Read the model definition and answer for the solid it produces. Units are mm, in the model's axes. Face numbers are marked on the shaded views. A direction names the side the tool comes from. Give positions to 0.01 mm unless a question says otherwise; leave off trailing zeros. Order: outer loops, then holes, each group sorted by start corner. A loop starts at its lowest first (then second) coordinate and runs counter-clockwise, first axis right, second up. Notation, with made-up numbers: M 16.5,70 L 36.5,70 A12 cw 36.5,79 Z; hole C 74,37 d6. An arc over 180 degrees is marked long. One line per item, written item: value.
Autodesk Inventor part; units mm, degrees
ref_plane "YZ Plane" through (0, 0, 0) normal (1, 0, 0) x (0, 1, 0)
ref_plane "XZ Plane" through (0, 0, 0) normal (0, 1, 0) x (-1, 0, 0)
ref_plane "XY Plane" through (0, 0, 0) normal (0, 0, 1) x (1, 0, 0)
sketch "Boceto1" plane through (0, 0, 0) normal (0, 1, 0) x (-1, 0, 0)
  line L0 (0, 0) -> (640, 0)
  line L1 (640, 0) -> (640, 1009)
  line L2 (640, 1009) -> (0, 1009)
  line L3 (0, 1009) -> (0, 0)
  dimension "d0" = 640
  dimension "d1" = 1009
extrude "Extrusión1" add sketch "Boceto1" along normal blind 1147
sketch "Boceto2" plane through (0, 1147, 0) normal (0, 1, 0) x (1, 0, 0)
  line L0 (-640, 0) -> (-640, -1009) construction
  line L1 (-640, -1009) -> (0, -1009) construction
  line L2 (0, -1009) -> (0, 0) construction
  line L3 (0, 0) -> (-640, 0) construction
  line L4 (-640, 0) -> (-640, -1009) construction
  line L5 (-640, -1009) -> (-640, -504.5) construction
  line L6 (0, -1009) -> (0, 0) construction
  line L7 (-640, -504.5) -> (0, -504.5) construction
  line L8 (0, -504.5) -> (0, -434.5) construction
  line L9 (0, -434.5) -> (-640, -434.5) construction
  line L10 (-640, -434.5) -> (-640, -504.5) construction
  line L11 (0, -434.5) -> (-640, -434.5)
  line L12 (-640, -434.5) -> (-640, -504.5)
  line L13 (-640, -504.5) -> (0, -504.5)
  line L14 (0, -504.5) -> (0, -434.5)
  dimension "d4" = 504.5
  dimension "d5" = 70
  dimension "d6" = 70
extrude "Extrusión2" add sketch "Boceto2" along normal blind 633
sketch "Boceto3" plane through (0, 1147, 0) normal (0, 1, 0) x (1, 0, 0)
  line L0 (-640, -434.5) -> (0, -434.5) construction
  line L1 (0, -434.5) -> (0, 0) construction
  line L2 (0, 0) -> (-640, 0) construction
  line L3 (-640, 0) -> (-640, -434.5) construction
  line L4 (0, -434.5) -> (0, 0) construction
  line L5 (0, -434.5) -> (-160, -434.5) construction
  line L6 (0, -434.5) -> (-640, -434.5) construction
  line L7 (-640, -434.5) -> (-640, -504.5) construction
  line L8 (-640, -434.5) -> (-480, -434.5) construction
  line L9 (-480, -434.5) -> (-160, -434.5)
  line L10 (-160, -434.5) -> (-160, -134.5)
  line L11 (-160, -134.5) -> (-480, -134.5)
  line L12 (-480, -134.5) -> (-480, -434.5)
  dimension "d9" = 160
  dimension "d10" = 160
  dimension "d11" = 300
extrude "Extrusión3" add sketch "Boceto3" along normal blind 53
sketch "Boceto4" plane through (0, 1200, 0) normal (0, 1, 0) x (1, 0, 0)
  line L0 (-160, -434.5) -> (-480, -434.5) construction
  line L1 (-160, -434.5) -> (-160, -134.5) construction
  line L2 (-160, -134.5) -> (-480, -134.5) construction
  line L3 (-480, -134.5) -> (-480, -434.5) construction
  line L4 (0, -434.5) -> (-640, -434.5) construction
  line L5 (-320, -434.5) -> (-320, -309.5) construction
  circle A0 centre (-320, -309.5) radius 30 construction
  line L6 (-320, -309.5) -> (-395, -309.5) construction
  line L7 (-395, -309.5) -> (-395, -339.5) construction
  line L8 (-395, -339.5) -> (-320, -339.5) construction
  line L9 (-320, -339.5) -> (-320, -309.5) construction
  line L10 (-395, -339.5) -> (-245, -339.5)
  line L11 (-245, -339.5) -> (-245, -279.5)
  line L12 (-245, -279.5) -> (-395, -279.5)
  line L13 (-395, -279.5) -> (-395, -339.5)
  point P0 (0, 0)
  dimension "d14" = 125
  dimension "d15" = 60
  dimension "d16" = 75
  dimension "d17" = 30
  dimension "d18" = 150
  dimension "d19" = 60
extrude "Extrusión4" add sketch "Boceto4" along normal blind 20
sketch "Boceto5" plane through (0, 1220, 0) normal (0, 1, 0) x (1, 0, 0)
  line L0 (-245, -279.5) -> (-395, -279.5) construction
  line L1 (-395, -279.5) -> (-395, -339.5) construction
  line L2 (-395, -339.5) -> (-245, -339.5) construction
  line L3 (-245, -339.5) -> (-245, -279.5) construction
  circle A0 centre (-320, -309.5) radius 30 construction
  line L4 (-320, -309.5) -> (-352, -309.5) construction
  line L5 (-352, -309.5) -> (-288, -309.5) construction
  line L6 (-395, -339.5) -> (-245, -339.5)
  line L7 (-352, -339.5) -> (-395, -339.5)
  line L8 (-395, -339.5) -> (-395, -279.5)
  line L9 (-395, -279.5) -> (-352, -279.5)
  line L10 (-352, -279.5) -> (-352, -339.5)
  line L11 (-245, -279.5) -> (-245, -339.5)
  line L12 (-395, -279.5) -> (-245, -279.5)
  line L13 (-245, -339.5) -> (-288, -339.5)
  line L14 (-288, -339.5) -> (-288, -279.5)
  line L15 (-288, -279.5) -> (-245, -279.5)
  line L16 (-245, -279.5) -> (-245, -339.5)
  point P0 (0, 0)
  dimension "d22" = 60
  dimension "d23" = 32
  dimension "d24" = 64
extrude "Extrusión5" add sketch "Boceto5" along normal blind 35 contours L8 L9 L10 L6 | L14 L12 L11 L6
chamfer "Chaflán1" distance 20 angle 45 1 edges at (-395, 1255, 309.5)
sketch "Boceto6" plane through (0, 0, 0) normal (0, -1, 0) x (1, 0, 0)
  line L0 (-640, 0) -> (-640, 1009) construction
  line L1 (0, 0) -> (-640, 0) construction
  line L2 (0, 1009) -> (0, 0) construction
  line L3 (-640, 1009) -> (0, 1009) construction
  line L4 (-640, 1009) -> (0, 1009)
  line L5 (0, 1009) -> (300, 1009)
  line L6 (300, 1009) -> (300, 405)
  line L7 (300, 405) -> (0, 405)
  line L8 (0, 405) -> (0, 1009)
  dimension "d30" = 300
  dimension "d31" = 604
extrude "Extrusión6" add sketch "Boceto6" against normal blind 1133
sketch "Boceto7" plane through (0, 1220, 0) normal (0, 1, 0) x (1, 0, 0)
  line L0 (-352, -279.5) -> (-352, -339.5)
  line L1 (-352, -339.5) -> (-288, -339.5)
  line L2 (-288, -339.5) -> (-288, -279.5)
  line L3 (-288, -279.5) -> (-352, -279.5)
  circle A0 centre (-320, -309.5) radius 30
  point P0 (0, 0)
  dimension "d34" = 60
  dimension "d35" = 32
properties part number "CMM"
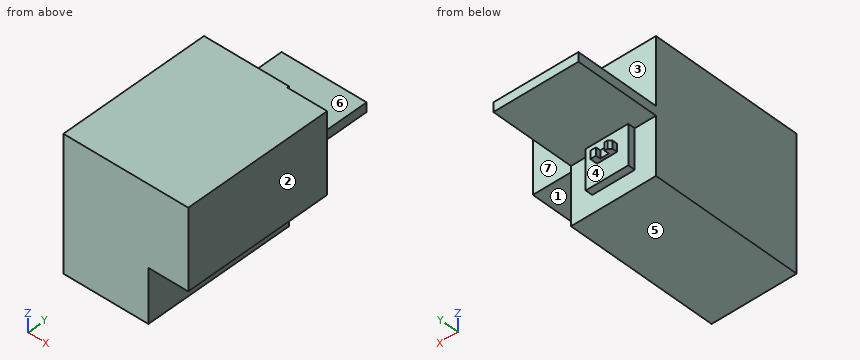
1) Find section D-D, the plane z = 364. Write down the section's boundary in (x, y), plus the area to 3 significant figures.
Reported:
outline: M -640,0 L 0,0 L 0,1147 L -160,1147 L -160,1200 L -480,1200 L -480,1147 L -640,1147 Z
area: 751,000 mm^2
2) Which of the six approach directions +Z, -Z, +X, -X, +Y, -Y give full straight-line access (tool end or side, diameter ignored) to the marked faces 1, 2 and 3?
Reported:
face 1: -Z, +X, +Y, -Y
face 2: +Z, -Z, +X, +Y, -Y
face 3: +Z, +X, -X, +Y
3) Find section A-A, the plane z = 624.5. Write down the section's boundary in (x, y), plus the area to 3 significant figures.
Reported:
outline: M -640,0 L 300,0 L 300,1133 L 0,1133 L 0,1147 L -640,1147 Z
area: 1,070,000 mm^2
4) Each of these flat-tipped pins is pushed along its axis until it touches: pin 1 Ø8 at (x, y) = (123.5, 208) entering from -Z; pin 2 Ø21.5 at (x, z) = (-257.5, 301) entering from +Y; pin 3 Ø1.5 at (y, z) = (1495, 451) entering from +X. Where does it stop, or does it pass through?
Reported:
pin 1: stops at z = 405
pin 2: stops at y = 1255
pin 3: stops at x = 0
5) Find section B-B, the plane y = 757. Write down the section's boundary in (x, z).
Reported:
outline: M -640,0 L 0,0 L 0,405 L 300,405 L 300,1009 L -640,1009 Z
6) Find section C-C, the plane x = -32.5. Write down the section's boundary in (y, z).
Reported:
outline: M 0,0 L 1147,0 L 1147,434.5 L 1780,434.5 L 1780,504.5 L 1147,504.5 L 1147,1009 L 0,1009 Z
7) Consider probe 1 along Z at (x, y) = (-74, 1160.5); probe 2 along Y at (x, z) = (-162, 660.5); probe 3 along Y at (x, z) = (-340, 250). Determine where each line is inside the solid, lowest interval first.
Reported:
probe 1: z = 434.5 to 504.5
probe 2: y = 0 to 1147
probe 3: y = 0 to 1200
8) Determine the mould class of the marked faces 4, 5, 6 and 7 for opening direction Z: +Z half, -Z half, draft (parallel to the pull), parting line (faces both ways), or undercut.
Reported:
face 4: undercut
face 5: -Z half
face 6: +Z half
face 7: draft
